Source: CAD feature listing. Evaluate the final solid. Frame: model axes, mm. A direction names the side the tool comes from. Coordinates: 2 decimals unless noted, no trailing zeros. Order: outer loops, then holes, each group sorted by start corner. A loop starts at its lowest first (then second) coordinate and runs counter-clockwise, first axis right, second up. Notation, with made-up numbers: (30.25, 47.5) -> (36.25, 47.5) arc R35 cw to (36.25, 85.5) -> close; hole circle Ø6 at (-16, 40.5). An arc over 180 degrees is marked (long way). Put each result on its own line as item: value.
from build123d import *

# Parameters (mm, degrees)
ESQUISSE1_R        = 2.8
BOSS_EXTRU_1_DEPTH = 122


with BuildPart() as part:
    # Esquisse1 → Boss.-Extru.1 (new body)
    with BuildSketch(Plane.XY):
        Polygon((-12, 5), (-12, -5), (12, -5), (12, 5), (8, 5), (8, -1), (5, -1), (5, 5), (-5, 5), (-5, -1), (-8, -1), (-8, 5), align=None)
        Circle(ESQUISSE1_R, mode=Mode.SUBTRACT)
    extrude(amount=BOSS_EXTRU_1_DEPTH)


solid = part.part
1. Pull-direction query (Y, two-part tool) for faces 1 (the flat face through (0, -5, 60)), 2 (the flat face through (-12, 0, 60)), 3 (the flat face through (10, 5, 60)), 4 (the cylindrical face through (-2.8, 0.1, 60.1)); classes: pulls with the +Y half, pulls with the -Y half, needs draft (parallel to the pull), parting line crosses it, or undercut.
Numbers:
face 1: pulls with the -Y half
face 2: needs draft
face 3: pulls with the +Y half
face 4: undercut
2. Set-up query: faces 5 (the flat face through (5, 2, 60)), 6 (the flat face through (-10, 5, 60)). Return all of +Z, -Z, +X, -X, +Y, -Y with unobstructed straight access to the full face (end or side cutting, diameter ignored); none if empty.
Numbers:
face 5: +Z, -Z, +Y
face 6: +Z, -Z, +X, -X, +Y
3. Cut plane C-C on z = 24. Output: boundary loops of the cut face in (x, y), plus the area to 3 significant figures.
Numbers:
outline: (-12, -5) -> (12, -5) -> (12, 5) -> (8, 5) -> (8, -1) -> (5, -1) -> (5, 5) -> (-5, 5) -> (-5, -1) -> (-8, -1) -> (-8, 5) -> (-12, 5) -> close; hole circle Ø5.6 at (0, 0)
area: 179 mm2
4. First-contact query: pin 1 (1.5 mm diameter, centred on x = 6.5, z = 50, fed in from +Y). Flat tip, straight axial feed; report the tip coordinate or a pass-through.
Numbers:
pin 1: stops at y = -1
5. Cut plane B-B on y = 0. Output: boundary loops of the cut face in (x, z), plus the area to 3 significant figures.
Numbers:
outline: (-12, 0) -> (-8, 0) -> (-8, 122) -> (-12, 122) -> close; (-5, 0) -> (-2.8, 0) -> (-2.8, 122) -> (-5, 122) -> close; (2.8, 0) -> (5, 0) -> (5, 122) -> (2.8, 122) -> close; (8, 0) -> (12, 0) -> (12, 122) -> (8, 122) -> close
area: 1,510 mm2
6. Ray query, line 1 along Y through (x, z) = (0, 56.5); line 2 along X through (y, z) = (3, 14); line 3 along X through (y, z) = (1, 47.5). Return the intervals inside material, ascending.
Numbers:
line 1: y = -5 to -2.8, 2.8 to 5
line 2: x = -12 to -8, -5 to 5, 8 to 12
line 3: x = -12 to -8, -5 to -2.62, 2.62 to 5, 8 to 12
7. Cut plane A-A on x = 0. Output: boundary loops of the cut face in (y, z).
Numbers:
outline: (-5, 0) -> (-2.8, 0) -> (-2.8, 122) -> (-5, 122) -> close; (2.8, 0) -> (5, 0) -> (5, 122) -> (2.8, 122) -> close
